Can you work these out from the model? Positions are in its coordinate system, mm. Face numbers are marked on the shaded views. A direction names the side the tool comes from. Coordinates: 2 decimals unless noted, no trailing zeros. Order: outer loops, then holes, each group sorted by start corner. A loop starts at its lowest first (then second) coordinate and runs counter-clockwise, first axis right, second up. Notation, with made-up numbers: M -39,-32 L 0,-32 A19 ccw 0,-12 Z; hole C 30.5,45 d9. An arc over 180 degrees is marked long. Answer as CSV lines item,"result". Start each with the question number.
1. If we section it at B-B (z = -163.5): List the corners of the cut face in (x, y) for me.
2. If we section it at A-A (y = 103.5): List the corners of the cut face in (x, z) for me.
3. I need wall thicknesses on line 1 along Z through (x, y) = (-144.5, 85.5); line 2 along X through (y, z) = (163, -84.5); line 3 along Y through (x, z) = (3, -349.15). Which ranges of each line are inside material? Lowest first, please. Write a range as from..to.
4. If we mould it in two halves opening along X, with no side actions, what happens to the marked faces 3, 4 and 5? For each: released by +X, released by -X, zero draft, split by the parting line, or undercut.
5. If we section it at D-D (x = -125): List the corners of the cut face in (y, z) for me.
6. If we section it at C-C (y = 40): List the corners of the cut face in (x, z) for me, plus the area to 3 significant figures.
7. Will these pins go through, and if not, where does the flat tip stop? pin 1 (5 mm diameter, centred on x = -41, z = -63, fed in from -Y); pin 2 (2 mm diameter, centred on x = 120.5, z = 28.5, fed in from +Y); pin 3 (18 mm diameter, centred on x = 3, y = 40, fed in from -Z).
8. On a 3-axis mill with a long thin cutter (end or side, diameter ignored), from which of +Z, -Z, +X, -X, +Y, -Y can I reach the whole of each face in a straight line? I mean the marked faces 1 and 2. Say none if no direction works.
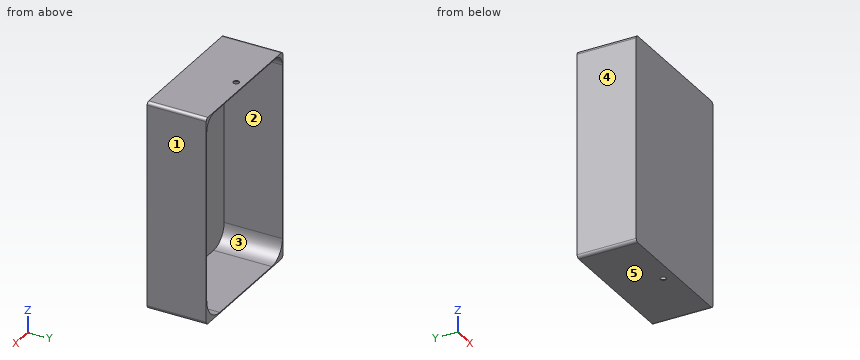
Autodesk Inventor part; units mm, degrees
ref_plane "YZ Plane" through (0, 0, 0) normal (1, 0, 0) x (0, 1, 0)
ref_plane "XZ Plane" through (0, 0, 0) normal (0, 1, 0) x (-1, 0, 0)
ref_plane "XY Plane" through (0, 0, 0) normal (0, 0, 1) x (1, 0, 0)
sketch "Sketch1" plane through (0, 0, 0) normal (0, 1, 0) x (-1, 0, 0)
  line L0 (230, 350) -> (-230, 350)
  line L1 (-230, 350) -> (-230, -350)
  line L2 (-230, -350) -> (230, -350)
  line L3 (230, -350) -> (230, 350)
  line L4 (230, 350) -> (-230, -350) construction
  line L5 (-230, 350) -> (230, -350) construction
  line L6 (227, 347) -> (-227, 347)
  line L7 (-227, 347) -> (-227, -347)
  line L8 (-227, -347) -> (227, -347)
  line L9 (227, -347) -> (227, 347)
  line L10 (227, 347) -> (-227, -347) construction
  line L11 (-227, 347) -> (227, -347) construction
  point P0 (0, 0)
  dimension "d0" = 460
  dimension "d1" = 700
  dimension "d2" = 454
  dimension "d3" = 694
extrude "Extrusion1" add sketch "Sketch1" along normal blind 3 contours L9 L8 L7 L6
extrude "Extrusion2" add sketch "Sketch1" along normal blind 200
sketch "Sketch2" plane through (-230, 0, 350) normal (0, 0, 1) x (1, 0, 0)
  line L0 (0, 0) -> (460, 0)
  line L1 (0, 0) -> (0, 200)
  point P0 (230, 0)
  point P1 (227, 170)
  dimension "d15" = 170
  dimension "d16" = 227
hole "Hole1" at (-3, 170, 350) direction (0, 0, -1) diameter 20 depth 3 tip angle 118
sketch "Sketch3" plane through (230, 0, -350) normal (0, 0, -1) x (-1, 0, 0)
  line L0 (0, 0) -> (0, 200)
  line L1 (0, 0) -> (460, 0)
  point P0 (230, 0)
  point P1 (227, 40)
  dimension "d24" = 227
  dimension "d25" = 40
hole "Hole2" at (3, 40, -350) direction (0, 0, 1) diameter 20 depth 3 tip angle 118
fillet "Fillet1" radius 10 4 edges at (230, 100, 350) (230, 100, -350) (-230, 100, 350) (-230, 100, -350)
fillet "Fillet2" radius 41.7 1 edges at (-227, 101.5, 347)
fillet "Fillet3" radius 63.3 1 edges at (-227, 101.5, -347)
fillet "Fillet4" radius 78.1 1 edges at (227, 101.5, -347)
fillet "Fillet5" radius 43.7 1 edges at (227, 101.5, 347)
properties part number "Ammonia Filter Tub"
Solved:
1,outline,"M -230,0 L 230,0 L 230,200 L 227,200 L 227,3 L -227,3 L -227,200 L -230,200 Z"
2,outline,"M -230,-340 A10 ccw -220,-350 L 220,-350 A10 ccw 230,-340 L 230,340 A10 ccw 220,350 L -220,350 A10 ccw -230,340 Z; hole M -227,-283.7 A63.3 ccw -163.7,-347 L 148.9,-347 A78.1 ccw 227,-268.9 L 227,303.3 A43.7 ccw 183.3,347 L -185.3,347 A41.7 ccw -227,305.3 Z"
3,line 1,"-350..-347, 347..350"
3,line 2,"-230..-227, 227..230"
3,line 3,"0..30, 50..200"
4,face 3,"undercut"
4,face 4,"released by -X"
4,face 5,"zero draft"
5,outline,"M 0,-350 L 200,-350 L 200,-347 L 3,-347 L 3,347 L 200,347 L 200,350 L 0,350 Z"
6,outline,"M -230,-340 A10 ccw -220,-350 L -7,-350 L -7,-347 L -163.7,-347 A63.3 cw -227,-283.7 L -227,305.3 A41.7 cw -185.3,347 L 183.3,347 A43.7 cw 227,303.3 L 227,-268.9 A78.1 cw 148.9,-347 L 13,-347 L 13,-350 L 220,-350 A10 ccw 230,-340 L 230,340 A10 ccw 220,350 L -220,350 A10 ccw -230,340 Z"
6,area,"9,730 mm²"
7,pin 1,"y = 0"
7,pin 2,"y = 3"
7,pin 3,"z = 347"
8,face 1,"+Z, -Z, +X, +Y, -Y"
8,face 2,"+Y"
